Can you work these out from the model? Positions are in its coordinate system, mm. Face numbers are marked on the shaded views. A direction names the side the tool comes from. Round coordinates to 2 decimals unless told otherwise and drop trailing zeros. Write each loop counter-clockwise with the first axis right and the second up, starting at its lowest first coordinate (ties: lowest second). Pieces come first, ordered by that corner, then holes.
Q1. For the marked faces 1 and 2, which set-ups out of +Z, -Z, +X, -X, +Y, -Y let a thin tool reach every point of the face, with its end or its side?
Q2. If we section it at A-A (x = 10.25): Please give me the cut outline in (y, z), plus the area to 3 significant figures.
Q3. I'm going to push flat-ended pins straight in: pin 1 Ø2 at (x, y) = (8, 0) entering from +Z; pin 2 Ø1.5 at (y, z) = (2, -1) entering from +X. Where does each tip first touch, or does it pass through?
Q4. Please list where these lines run through material, in increasing order: line 1 along X through (y, z) = (2, 0.5); line 2 along Y through (x, z) = (1.75, 1); line 3 along Y through (x, z) = (1, -1.5).
Autodesk Inventor part; units mm, degrees
ref_plane "Work Plane2" through (2.032, 0, 0) normal (0, 1, 0) x (1, 0, 0)
ref_plane "YZ Plane" through (0, 0, 0) normal (1, 0, 0) x (0, 1, 0)
ref_plane "XZ Plane" through (0, 0, 0) normal (0, 1, 0) x (-1, 0, 0)
sketch "Sketch1" plane through (0, 0, 0) normal (0, 0, 1) x (1, 0, 0)
  line L0 (2.6924, 0) -> (12.7, 0)
  line L1 (12.7, 0) -> (12.7, 1.7526)
  line L2 (12.7, 1.7526) -> (2.1082, 1.7526)
  line L3 (0.5596, 3.0988) -> (0, 3.0988)
  line L4 (-2.54, 0) -> (15.24, 0)
  line L5 (0, -0.6198) -> (0, 3.7186)
  line L6 (0, 2.2098) -> (2.0648, 1.1803)
  line L7 (2.0648, 1.1803) -> (2.6924, 0)
  line L8 (2.1082, 1.7526) -> (0.5596, 3.0988)
  line L9 (0, 3.0988) -> (0, 2.2098)
  dimension "d2" = 3.5052
  dimension "d3" = 6.1976
  dimension "d4" = 2.6924
  dimension "d5" = 4.4196
  dimension "d6" = 26.5
  dimension "d7" = 62
  dimension "d13" = 41
  dimension "d14" = 2.1082
  dimension "d15" = 12.7
revolve "Body" add sketch "Sketch1" angle 360 about axis through (2.6924, 0, 0) along (1, 0, 0) contours L7 L6 L5 L3 L8 L2 L1 L0
sketch "Sketch2" plane through (0, 0, 0) normal (-1, 0, 0) x (0, 0, 1)
  line L0 (0, -4.3383) -> (0, 4.3383)
  line L1 (-4.3383, 0) -> (4.3383, 0)
  line L2 (0, 2.2098) -> (0, 0) construction
  line L3 (0, 0) -> (2.2098, 0) construction
  arc A0 (0.7366, 0) -> (0, 0.7366) centre (0, 0) ccw
  line L4 (0, 0) -> (0.7947, 0.7947) construction
  arc A1 (1.1049, 0) -> (0, 1.1049) centre (0, 0) ccw construction
  line L5 (0.3683, 2.1789) -> (0.3131, 1.0596)
  line L6 (2.1789, 0.3683) -> (1.0596, 0.3131)
  arc A2 (0.3131, 1.0596) -> (1.0596, 0.3131) centre (1.0245, 1.0245) ccw
  arc A3 (2.2098, 0) -> (2.1789, 0.3683) centre (0, 0) ccw
  arc A4 (0.3683, 2.1789) -> (0, 2.2098) centre (0, 0) ccw
  arc A5 (2.1789, 0.3683) -> (0.3683, 2.1789) centre (0, 0) ccw
  line L7 (0.3683, -2.1789) -> (0.3131, -1.0596)
  line L8 (2.1789, -0.3683) -> (1.0596, -0.3131)
  arc A6 (1.0596, -0.3131) -> (0.3131, -1.0596) centre (1.0245, -1.0245) ccw
  arc A7 (2.1789, -0.3683) -> (2.2098, 0) centre (0, 0) ccw
  arc A8 (0, -2.2098) -> (0.3683, -2.1789) centre (0, 0) ccw
  arc A9 (0.3683, -2.1789) -> (2.1789, -0.3683) centre (0, 0) ccw
  line L9 (-0.3683, 2.1789) -> (-0.3131, 1.0596)
  line L10 (-2.1789, 0.3683) -> (-1.0596, 0.3131)
  arc A10 (-1.0596, 0.3131) -> (-0.3131, 1.0596) centre (-1.0245, 1.0245) ccw
  arc A11 (-2.1789, 0.3683) -> (-2.2098, 0) centre (0, 0) ccw
  arc A12 (0, 2.2098) -> (-0.3683, 2.1789) centre (0, 0) ccw
  arc A13 (-0.3683, 2.1789) -> (-2.1789, 0.3683) centre (0, 0) ccw
  arc A14 (-2.1789, -0.3683) -> (-0.3683, -2.1789) centre (0, 0) ccw
  arc A15 (-0.3683, -2.1789) -> (0, -2.2098) centre (0, 0) ccw
  arc A16 (-2.2098, 0) -> (-2.1789, -0.3683) centre (0, 0) ccw
  line L11 (-2.1789, -0.3683) -> (-1.0596, -0.3131)
  arc A17 (-0.3131, -1.0596) -> (-1.0596, -0.3131) centre (-1.0245, -1.0245) ccw
  line L12 (-0.3683, -2.1789) -> (-0.3131, -1.0596)
  dimension "d18" = 45
  dimension "d19" = 1.4732
  dimension "d20" = 2.2098
  dimension "d21" = 4.4196
  dimension "d22" = 0.3683
extrude "Slot" add sketch "Sketch2" against normal up to next contours A2 L5 A5 L6 | L9 A10 L10 A13 | L7 A6 L8 A9 | A14 L11 A17 L12
fillet "Fillet1" radius 0.1473 4 edges at (0, 2.2098, 0) (0, 0, 2.2098) (0, -2.2098, 0) (0, 0, -2.2098)
thread "Thread"
chamfer "Chamfer1" distance 0.5953 distance2 0.5953 1 edges at (12.7, -1.7526, 0) measured on face at (12.7, -0.023, 0.3874)
ref_plane "Work Plane2" through (2.032, 0, 0) normal (0, 1, 0) x (1, 0, 0)
equation "\"d2\" = GD"
equation "\"d3\" = KOD"
equation "\"d4\" = INTI"
equation "\"d5\" = SDM"
equation "\"d13\" = 0.5 * SEWI"
equation "\"d14\" = KOH"
equation "\"d15\" = NLG"
equation "\"d19\" = 0.333333 * SDM"
equation "\"d20\" = 0.5 * SDM"
equation "\"d21\" = SDM"
equation "\"d22\" = 0.5 * SBR"
equation "\"d45\" = INTI"
equation "\"d25\" = 0.2 * SBR"
equation "\"d9\" = GEL"
equation "\"d11\" = -0.5 * SPD + 0.5 * GD"
equation "\"d12\" = GUL"
equation "\"GD\" = NND"
equation "\"NLG\" = 12.7"
equation "\"GEL\" = 8.60742"
equation "\"KOD\" = 6.1976"
equation "\"KOH\" = 2.1082"
equation "\"SDM\" = 4.4196"
equation "\"INTI\" = 2.6924"
equation "\"SBR\" = 0.7366"
equation "\"GUL\" = 0.75 * GAL"
equation "\"SPD\" = 2.31458"
equation "\"SEWI\" = 82deg"
equation "\"d0\" = NLG"
equation "\"d1\" = KOH"
equation "\"d17\" = SDM"
equation "\"TOA\" = 30deg"
equation "\"THREADDIA\" = 3.5052"
equation "\"BDM\" = NND"
equation "\"NND\" = 3.5052"
equation "\"GAL\" = 0.79375"
equation "\"GD1\" = SPD"
properties part number "ANSI B18.6.3 - 6-32 x 1/2, CRFCHMSTII(5)" material "Steel, Mild"
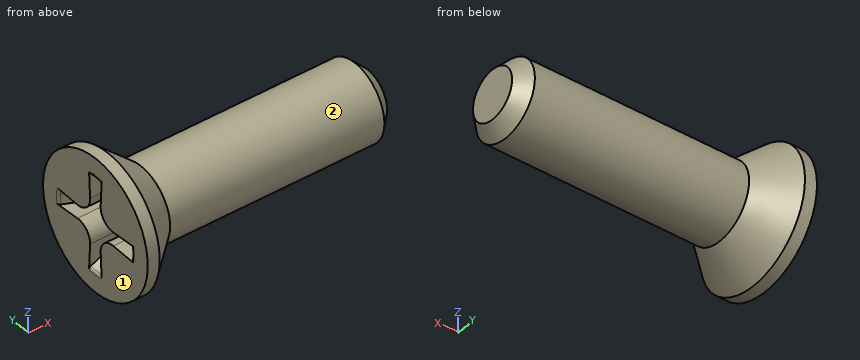
A:
1. face 1: +Z, -Z, -X, +Y, -Y
1. face 2: +X
2. outline: circle Ø3.51 at (0, 0)
2. area: 9.65 mm2
3. pin 1: stops at z = 1.75
3. pin 2: stops at x = 12.37
4. line 1: x = 0 to 1.75
4. line 2: y = -1.81 to -0.31, 0.31 to 1.81
4. line 3: y = -2.26 to -0.33, 0.33 to 2.26
